from build123d import *
from OCP.BRepFilletAPI import BRepFilletAPI_MakeChamfer

# Parameters (mm, degrees)
BOSS_EXTRUDE1_DEPTH = 2
SKETCH2_R           = 9.35
CUT_EXTRUDE1_DEPTH  = 26.816661287
BOSS_EXTRUDE3_START = 3
BOSS_EXTRUDE3_DEPTH = 3
CHAMFER1_SIZE       = 3
CHAMFER1_SIZE2      = 0.5
SKETCH5_W           = 15
SKETCH5_H           = 12
CUT_EXTRUDE3_DEPTH  = 1
CHAMFER2_SIZE       = 2
CHAMFER2_SIZE_2     = 1
SKETCH7_R           = 0.75
SKETCH7_R_2         = 1.6
CUT_EXTRUDE4_DEPTH  = 27.220221204


with BuildPart() as part:
    # Sketch1 → Boss-Extrude1 (new body)
    with BuildSketch(Plane(origin=(0, 0, 0), x_dir=(1, 0, 0), z_dir=(0, 1, 0))):
        with BuildLine():
            Line((10, -12.5), (-10, -12.5))
            ThreePointArc((-10, -12.5), (-22.5, 0), (-10, 12.5))
            Line((-10, 12.5), (10, 12.5))
            ThreePointArc((10, 12.5), (22.5, 0), (10, -12.5))
        make_face()
    extrude(amount=BOSS_EXTRUDE1_DEPTH)

    # Sketch2 → Cut-Extrude1 (cut, through all)
    with BuildSketch(Plane(origin=(0, 2, 0), x_dir=(1, 0, 0), z_dir=(0, 1, 0))):
        with Locations(Location((10, 0, 0), (0, 0, 270))):
            Circle(SKETCH2_R)
        with Locations(Location((-10, 0, 0), (0, 0, 90))):
            Circle(SKETCH2_R)
    extrude(amount=-CUT_EXTRUDE1_DEPTH, mode=Mode.SUBTRACT)

    # Sketch3 → Boss-Extrude3 (add)
    with BuildSketch(Plane.XZ.offset(BOSS_EXTRUDE3_START)):
        with BuildLine():
            Line((-10, -12.5), (10, -12.5))
            ThreePointArc((10, -12.5), (22.5, 0), (10, 12.5))
            Line((10, 12.5), (-10, 12.5))
            ThreePointArc((-10, 12.5), (-22.5, 0), (-10, -12.5))
        make_face()
        with BuildLine():
            Line((-10, -11.5), (10, -11.5))
            ThreePointArc((10, -11.5), (21.5, 0), (10, 11.5))
            Line((10, 11.5), (-10, 11.5))
            ThreePointArc((-10, 11.5), (-21.5, 0), (-10, -11.5))
        make_face(mode=Mode.SUBTRACT)
    extrude(amount=-BOSS_EXTRUDE3_DEPTH)

    # Chamfer1: one chamfer whose edges measure the first distance from different faces: ONE call of the kernel's chamfer builder (chamfer() names one face for all edges)
    chamfer1_edges_1 = [part.edges().sort_by_distance(p)[0] for p in [
        (22.5, -3, 0),
    ]]
    chamfer1_side_1 = [part.faces().sort_by_distance(p)[0] for p in [
        (22.5, -0.5, 0),
    ]]
    chamfer1_edges_2 = [part.edges().sort_by_distance(p)[0] for p in [
        (0, -3, 12.5),
    ]]
    chamfer1_side_2 = [part.faces().sort_by_distance(p)[0] for p in [
        (0, -0.5, 12.5),
    ]]
    chamfer1_edges_3 = [part.edges().sort_by_distance(p)[0] for p in [
        (-22.5, -3, 0),
    ]]
    chamfer1_side_3 = [part.faces().sort_by_distance(p)[0] for p in [
        (-22.5, -0.5, 0),
    ]]
    chamfer1_edges_4 = [part.edges().sort_by_distance(p)[0] for p in [
        (0, -3, -12.5),
    ]]
    chamfer1_side_4 = [part.faces().sort_by_distance(p)[0] for p in [
        (0, -0.5, -12.5),
    ]]
    chamfer1 = BRepFilletAPI_MakeChamfer(part.part.solid().wrapped)
    for e in chamfer1_edges_1:
        chamfer1.Add(CHAMFER1_SIZE, CHAMFER1_SIZE2, e.wrapped, chamfer1_side_1[0].wrapped)  # the first distance lies on this face
    for e in chamfer1_edges_2:
        chamfer1.Add(CHAMFER1_SIZE, CHAMFER1_SIZE2, e.wrapped, chamfer1_side_2[0].wrapped)  # the first distance lies on this face
    for e in chamfer1_edges_3:
        chamfer1.Add(CHAMFER1_SIZE, CHAMFER1_SIZE2, e.wrapped, chamfer1_side_3[0].wrapped)  # the first distance lies on this face
    for e in chamfer1_edges_4:
        chamfer1.Add(CHAMFER1_SIZE, CHAMFER1_SIZE2, e.wrapped, chamfer1_side_4[0].wrapped)  # the first distance lies on this face
    add(Compound.cast(chamfer1.Shape()), mode=Mode.REPLACE)

    # Sketch5 → Cut-Extrude3 (cut)
    with BuildSketch(Plane.XZ):
        Rectangle(SKETCH5_W, SKETCH5_H)
    extrude(amount=-CUT_EXTRUDE3_DEPTH, mode=Mode.SUBTRACT)

    # Chamfer2
    chamfer2_edges_1 = [part.edges().sort_by_distance(p)[0] for p in [
        (0, 1, -6),
    ]]
    chamfer2_side_1 = [part.faces().sort_by_distance(p)[0] for p in [
        (0, 1, -5.98),
    ]]
    chamfer2_edges_2 = [part.edges().sort_by_distance(p)[0] for p in [
        (0, 1, 6),
    ]]
    chamfer2_side_2 = [part.faces().sort_by_distance(p)[0] for p in [
        (0, 0.98, 6),
    ]]
    chamfer2 = BRepFilletAPI_MakeChamfer(part.part.solid().wrapped)
    for e in chamfer2_edges_1:
        chamfer2.Add(CHAMFER2_SIZE - 0.0001, CHAMFER2_SIZE_2 - 0.0001, e.wrapped, chamfer2_side_1[0].wrapped)
    for e in chamfer2_edges_2:
        chamfer2.Add(CHAMFER2_SIZE_2 - 0.0001, CHAMFER2_SIZE - 0.0001, e.wrapped, chamfer2_side_2[0].wrapped)
    add(Compound.cast(chamfer2.Shape()), mode=Mode.REPLACE)  # a hair under: the kernel refuses the full size

    # Sketch7 → Cut-Extrude4 (cut, through all)
    with BuildSketch(Plane(origin=(0, 2, 0), x_dir=(1, 0, 0), z_dir=(0, 1, 0))):
        with Locations(Location((-4, -9.5, 0), (0, 0, 270))):
            Circle(SKETCH7_R)
        with Locations(Location((0, -9, 0), (0, 0, 270))):
            Circle(SKETCH7_R_2)
        with Locations(Location((0, 9, 0), (0, 0, 270))):
            Circle(SKETCH7_R_2)
    extrude(amount=-CUT_EXTRUDE4_DEPTH, mode=Mode.SUBTRACT)


solid = part.part
The listing builds one solid part. Answer for the finished solid, in the listing's coordinates (mm). A direction names the side the tool comes from. Round coordinates to 2 decimals unless told otherwise and drop trailing zeros. Write each loop counter-clockwise with the first axis right and the second up, starting at its lowest first coordinate (ties: lowest second). Pieces come first, ordered by that corner, then holes. Notation, with made-up numbers: M -39.75,21.5 L -34.75,21.5 A27 ccw -34.75,49.5 Z; hole C -23.75,-3 d2. An arc over 180 degrees is marked long. Write each question's results on one line, items separated by ' | '. Start each with the question number.
Item 1: The mould has two halves that part along X. Classify faces 3 (the conical face through (22.13, -2.19, -0.27)), 4 (the flat face through (0, 0.5, 5)), 5 (the flat face through (0, 1, -12.5)), 6 (the cylindrical face through (-19.27, 1.01, 1.22)): +X half, -X half, draft (parallel to the pull), parting line (faces both ways), or undercut.
Item 2: Find section B-B on y = -1.2. Write down the section's boundary in (x, z), and give its area (3 significant figures).
Item 3: Find section D-D on y = 1.55. Write down the section's boundary in (x, z).
Item 4: Given pin 1 Ø7 at (x, z) = (0.5, 3) entering from -Y; pin 2 Ø1.5 at (x, y) = (1, -1) entering from +Z; pin 3 Ø0.9 at (x, z) = (-0.5, 0.5) entering from -Y, each flat-ended and moving along its own axis, determine where each tip first touches the part or whether it passes through.
Item 5: Find section A-A on x = 0. Give the number of separate pieces and of enclosed holes in the cut face, and give its area (3 significant figures).
Item 6: Which of the six approach directions +Z, -Z, +X, -X, +Y, -Y give full straight-line access (tool end or side, diameter ignored) to faces 1 (the flat face through (0, 0.4, -5.2)), 2 (the cylindrical face through (22.497, 0.986, -0.275))?
Item 7: Find section C-C on x = 6. Write down the section's boundary in (y, z), and give its area (3 significant figures).
Item 8: Straight lines are drawn through the part: probe 1 along X at (y, z) = (1.2, 0); probe 2 along X at (y, z) = (0.85, 9.5); probe 3 along X at (y, z) = (0.5, 0). For each, find the intervals that lie inside material, in ascending order.
Answer block:
1) face 3: +X half | face 4: undercut | face 5: draft | face 6: undercut
2) outline: M -10,-12.3 L 10,-12.3 A12.3 ccw 10,12.3 L -10,12.3 A12.3 ccw Z; hole M -10,-11.5 L 10,-11.5 A11.5 ccw 10,11.5 L -10,11.5 A11.5 ccw Z | area: 91.8 mm²
3) outline: M -10,-12.5 L 10,-12.5 A12.5 ccw 10,12.5 L -10,12.5 A12.5 ccw Z; hole C -10,0 d18.7; hole C -4,9.5 d1.5; hole C 0,-9 d3.2; hole C 0,9 d3.2; hole C 10,0 d18.7
4) pin 1: stops at y = 0 | pin 2: stops at z = 12.46 | pin 3: stops at y = 1
5) separate pieces: 3 | enclosed holes: 0 | area: 31.7 mm²
6) face 1: -Y | face 2: +X, +Y, -Y
7) outline: M -3,-12 L 0,-12.5 L 2,-12.5 L 2,-8.45 L 0,-8.45 L 0,-11.5 L -3,-11.5 Z; M -3,11.5 L 0,11.5 L 0,8.45 L 2,8.45 L 2,12.5 L 0,12.5 L -3,12 Z | area: 20.7 mm²
8) probe 1: x = -22.5 to -19.35, -0.65 to 0.65, 19.35 to 22.5 | probe 2: x = -18.12 to -4.75, -3.25 to -1.52, 1.52 to 18.12 | probe 3: x = -22.5 to -19.35, 19.35 to 22.5
